from build123d import *

# Parameters (mm, degrees)
SKETCH1_R           = 8
BOSS_EXTRUDE1_DEPTH = 250
SKETCH2_R           = 5
BOSS_EXTRUDE2_DEPTH = 10
SKETCH3_R           = 5
BOSS_EXTRUDE3_DEPTH = 10
SKETCH4_R           = 4
BOSS_EXTRUDE4_DEPTH = 30


with BuildPart() as part:
    # Sketch1 → Boss-Extrude1 (new body)
    with BuildSketch(Plane.XY):
        Circle(SKETCH1_R)
    extrude(amount=BOSS_EXTRUDE1_DEPTH)

    # Sketch2 → Boss-Extrude2 (add)
    with BuildSketch(Plane.XY.offset(250)):
        Circle(SKETCH2_R)
    extrude(amount=BOSS_EXTRUDE2_DEPTH)

    # Sketch3 → Boss-Extrude3 (add)
    with BuildSketch(Plane(origin=(0, 0, 0), x_dir=(-1, 0, 0), z_dir=(0, 0, -1))):
        Circle(SKETCH3_R)
    extrude(amount=BOSS_EXTRUDE3_DEPTH)

    # Sketch4 → Boss-Extrude4 (add)
    with BuildSketch(Plane(origin=(0, 0, -10), x_dir=(-1, 0, 0), z_dir=(0, 0, -1))):
        Circle(SKETCH4_R)
    extrude(amount=BOSS_EXTRUDE4_DEPTH)


solid = part.part
Geometry check sheet. Reference: the model listing, model coordinates, mm. A direction names the side the tool comes from. Give positions to 0.01 mm unless a question says otherwise; leave off trailing zeros. Loops run counter-clockwise (first coordinate to the right, second up) from the corner with the lowest first, then second, coordinate; pieces in that order, holes last.
(1) Section check C-C on z = 108. Record the cut outline in (x, y), then the cut area to 3 significant figures.
From the geometry:
outline: circle Ø16 at (0, 0)
area: 201 mm2
(2) Thickness scan on L1, parallel to Z at x = -6.75, y = -1.5; L2, parallel to Z at x = 4.5, y = -0.5; L3, parallel to Y at x = -6.25, z = 35. Record the ranges inside material, lowest first.
From the geometry:
L1: z = 0 to 250
L2: z = -10 to 260
L3: y = -4.99 to 4.99
(3) Section check A-A on y = 0. Record the cut outline in (x, z).
From the geometry:
outline: (-8, 0) - (-5, 0) - (-5, -10) - (-4, -10) - (-4, -40) - (4, -40) - (4, -10) - (5, -10) - (5, 0) - (8, 0) - (8, 250) - (5, 250) - (5, 260) - (-5, 260) - (-5, 250) - (-8, 250) - close
(4) Set-up check for faces 1 (the cylindrical face through (-1.73, -7.81, 123.25)), 2 (the cylindrical face through (0.867, -3.905, -24.79)), 3 (the cylindrical face through (-1.08, -4.88, 254.93)): record each of +Z, -Z, +X, -X, +Y, -Y from which the full face is reachable in a straight line by a thin tool's end or side.
From the geometry:
face 1: +Z, -Z
face 2: -Z
face 3: +Z
(5) Depth check by flat-ended pin: pin 1 Ø1 at (x, z) = (4.5, 73) entering from -Y; pin 2 Ø4 at (x, z) = (3.5, 21) entering from +Y; pin 3 Ø3 at (x, y) = (-6, 6) entering from -Z; pin 4 Ø3 at (x, y) = (-1.5, 4.5) entering from -Z. Enter the tip coordinate at first touch or a pass-through.
From the geometry:
pin 1: stops at y = -6.93
pin 2: stops at y = 7.86
pin 3: stops at z = 0
pin 4: stops at z = -40
